```python
from build123d import *

# Parameters (mm, degrees)
SKETCH_1_R          = 2.1
SKETCH_1_W          = 192
SKETCH_1_H          = 64
EXTRUDE_1_DEPTH     = 8
SKETCH_3_W          = 8
SKETCH_3_H          = 8
CUT_EXTRUDE_1_DEPTH = 2


with BuildPart() as part:
    # Эскиз1 → Бобышка-Вытянуть1 (new body)
    with BuildSketch(Plane(origin=(0, 8, 0), x_dir=(1, 0, 0), z_dir=(0, 1, 0))):
        Polygon((109.289774647, 94.419345598), (109.289774647, -5.580654402), (93.289774647, -5.580654402), (93.289774647, 4.419345598), (-74.710225353, 4.419345598), (-74.710225353, -5.580654402), (-90.710225353, -5.580654402), (-90.710225353, 94.419345598), (-74.710225353, 94.419345598), (-74.710225353, 84.419345598), (93.289774647, 84.419345598), (93.289774647, 94.419345598), align=None)
        with Locations(Location((-82.710225353, 89.419345598, 0), (0, 0, 180))):
            Circle(SKETCH_1_R, mode=Mode.SUBTRACT)
        with Locations(Location((-82.710225353, -0.580654402, 0), (0, 0, 180))):
            Circle(SKETCH_1_R, mode=Mode.SUBTRACT)
        with Locations(Location((101.289774647, -0.580654402, 0), (0, 0, 180))):
            Circle(SKETCH_1_R, mode=Mode.SUBTRACT)
        with Locations(Location((101.289774647, 89.419345598, 0), (0, 0, 180))):
            Circle(SKETCH_1_R, mode=Mode.SUBTRACT)
        with Locations((9.289774647, 44.419345598)):
            Rectangle(SKETCH_1_W, SKETCH_1_H, mode=Mode.SUBTRACT)
    extrude(amount=EXTRUDE_1_DEPTH)

    # Эскиз3 → Вырез-Вытянуть1 (cut)
    with BuildSketch(Plane(origin=(0, 8, 0), x_dir=(1, 0, 0), z_dir=(0, 1, 0))):
        with Locations((-9.710225353, 8.419345598)):
            Rectangle(SKETCH_3_W, SKETCH_3_H)
    extrude(amount=CUT_EXTRUDE_1_DEPTH, mode=Mode.SUBTRACT)


solid = part.part
```
Model file for the job. Use its own axes, mm. A direction names the side the tool comes from. Give positions to 0.01 mm unless a question says otherwise; leave off trailing zeros. Order: outer loops, then holes, each group sorted by start corner. A loop starts at its lowest first (then second) coordinate and runs counter-clockwise, first axis right, second up.
1) Saw through at B-B, the plane x = -9.5. Write the cut outline in (y, z), then the cut area to 3 significant figures.
2) Mould opens along Z. For faces 4 (the flat face through (10, 12, -4.419)), 5 (the cylindrical face through (100.32, 11.94, -91.28)), 6 (the flat face through (105.29, 12, -44)), 7 (the flat face through (-74.71, 12, -89)) say: +Z half, -Z half, draft (parallel to the pull), parting line (faces both ways), or undercut.
3) Pin check, flat tips, straight feed: pin 1 (2.5 mm diameter, centred on x = -1.5, y = 13.5, fed in from -Z); pin 2 (2.5 mm diameter, centred on x = -8, y = 12.5, fed in from +Z); pin 3 (4 mm diameter, centred on x = -8, z = -8.5, fed in from -Y). Stop position of each tip, or through.
4) 3-axis set-ups, long thin cutter, end or side, ignore diameter. For faces 1 (the flat face through (-74.71, 12, 1)), 2 (the flat face through (93.29, 12, -89)), 3 (the flat face through (8, 12, -12.419)): which of +Z, -Z, +X, -X, +Y, -Y reach the whole face in a straight line?
5) Saw through at A-A, the plane z = -46. Write the cut outline in (x, y), then the cut area to 3 significant figures.
6) Saw through at C-C, the plane y = 13.25. Write the cut outline in (x, z).
7) Wall check: probe 1 along X at (y, z) = (12, -36); probe 2 along X at (y, z) = (10, -85); probe 3 along Z at (x, y) = (-52, 14). Give the ranges that are in metal, low to high.
Computed:
1. outline: (8, -84.42) - (16, -84.42) - (16, -76.42) - (8, -76.42) - close; (10, -12.42) - (16, -12.42) - (16, -4.42) - (10, -4.42) - close
1. area: 112 mm2
2. face 4: +Z half
2. face 5: undercut
2. face 6: undercut
2. face 7: draft
3. pin 1: stops at z = -84.42
3. pin 2: stops at z = -4.42
3. pin 3: stops at y = 10
4. face 1: +Z, +Y, -Y
4. face 2: -Z, +Y, -Y
4. face 3: +Y, -Y
5. outline: (-90.71, 8) - (-86.71, 8) - (-86.71, 16) - (-90.71, 16) - close; (105.29, 8) - (109.29, 8) - (109.29, 16) - (105.29, 16) - close
5. area: 64.0 mm2
6. outline: (-90.71, -94.42) - (-74.71, -94.42) - (-74.71, -84.42) - (93.29, -84.42) - (93.29, -94.42) - (109.29, -94.42) - (109.29, 5.58) - (93.29, 5.58) - (93.29, -4.42) - (-74.71, -4.42) - (-74.71, 5.58) - (-90.71, 5.58) - close; hole (-86.71, -76.42) - (105.29, -76.42) - (105.29, -12.42) - (-86.71, -12.42) - close; hole circle Ø4.2 at (-82.71, -89.42); hole circle Ø4.2 at (-82.71, 0.58); hole circle Ø4.2 at (101.29, -89.42); hole circle Ø4.2 at (101.29, 0.58)
7. probe 1: x = -90.71 to -86.71, 105.29 to 109.29
7. probe 2: x = -90.71 to -74.71, 93.29 to 109.29
7. probe 3: z = -84.42 to -76.42, -12.42 to -4.42
